```python
from build123d import *

# Parameters (mm, degrees)
SKETCH1_W                        = 63.5
SKETCH1_H                        = 12.7
BOSS_EXTRUDE1_DEPTH              = 50.8
F_25_0_1495_DIAMETER_HOLE1_D     = 3.7973
F_25_0_1495_DIAMETER_HOLE1_DEPTH = 12.7
F_25_0_1495_DIAMETER_HOLE1_TIP   = 1.140824014
F_7_0_201_DIAMETER_HOLE1_D       = 5.1054
F_7_0_201_DIAMETER_HOLE1_DEPTH   = 12.7
F_7_0_201_DIAMETER_HOLE1_TIP     = 1.533816902


with BuildPart() as part:
    # Sketch1 → Boss-Extrude1 (new body)
    with BuildSketch(Plane(origin=(0, 0, 0), x_dir=(1, 0, 0), z_dir=(0, 1, 0))):
        with Locations((31.75, 6.35)):
            Rectangle(SKETCH1_W, SKETCH1_H)
    extrude(amount=BOSS_EXTRUDE1_DEPTH)

    # #25 (0.1495) Diameter Hole1
    with Locations(Plane(origin=(0, 50.8, 0), x_dir=(1, 0, 0), z_dir=(0, 1, 0))):
        with Locations((6.35, 6.35), (57.15, 6.35)):
            Hole(F_25_0_1495_DIAMETER_HOLE1_D / 2, depth=F_25_0_1495_DIAMETER_HOLE1_DEPTH)
            with Locations((0, 0, -(F_25_0_1495_DIAMETER_HOLE1_DEPTH + F_25_0_1495_DIAMETER_HOLE1_TIP / 2))):  # 118° drill point
                Cone(0, F_25_0_1495_DIAMETER_HOLE1_D / 2, F_25_0_1495_DIAMETER_HOLE1_TIP, mode=Mode.SUBTRACT)

    # #7 (0.201) Diameter Hole1
    with Locations(Plane(origin=(0, 0, -12.7), x_dir=(-1, 0, 0), z_dir=(0, 0, -1))):
        with Locations((-22.225, 43.18), (-41.275, 43.18)):
            Hole(F_7_0_201_DIAMETER_HOLE1_D / 2, depth=F_7_0_201_DIAMETER_HOLE1_DEPTH)
            with Locations((0, 0, -(F_7_0_201_DIAMETER_HOLE1_DEPTH + F_7_0_201_DIAMETER_HOLE1_TIP / 2))):  # 118° drill point
                Cone(0, F_7_0_201_DIAMETER_HOLE1_D / 2, F_7_0_201_DIAMETER_HOLE1_TIP, mode=Mode.SUBTRACT)


solid = part.part
```
Model file for the job. Use its own axes, mm. Coordinates: 2 decimals unless noted, no trailing zeros. Write each loop counter-clockwise with the first axis right and the second up, starting at its lowest first coordinate (ties: lowest second). Pieces come first, ordered by that corner, then holes. Notation, with made-up numbers: (32, 75.25) - (44, 75.25) arc R23 ccw to (44, 102.25) - close; hole circle Ø6 at (-14, 2.25). An arc over 180 degrees is marked (long way). One line per question, with ' | ' between items. Start each with the question number.
Q1. Pull direction X, two halves, no side cores. Call faces 1 (the face through (55.34, 44.36, -6.92)), 2 (the face through (31, 25, -12.7)), 3 (the face through (7.857, 44.361, -5.195)), 4 (the face through (0, 25, -6)): pulls with the +X half, pulls with the -X half, needs draft (parallel to the pull), parting line crosses it, or undercut.
Q2. Drill centre lines: line 1 (X direction, y = 43.18, z = -8.75); line 2 (X direction, y = 45, z = -6.5); line 3 (Z direction, x = 57.15, y = 47.5). Where is each one in solid material? Low to high. Write a range as [from, to].
Q3. Pin check, flat tips, straight feed: pin 1 (3 mm diameter, centred on y = 16, z = -4, fed in from -X); pin 2 (2.5 mm diameter, centred on x = 6.35, z = -6.35, fed in from +Y); pin 3 (3 mm diameter, centred on x = 22.225, y = 43.18, fed in from -Z). Stop position of each tip, or through.
Q4. Cut at A-A, the plane y = 43.18. List the corners of the cut face in (x, z).
Answer below:
1) face 1: undercut | face 2: needs draft | face 3: undercut | face 4: pulls with the -X half
2) line 1: [0, 19.67], [24.78, 38.72], [43.83, 63.5] | line 2: [0, 4.46], [8.24, 20.44], [24.01, 39.49], [43.06, 55.26], [59.04, 63.5] | line 3: [-12.7, -8.25], [-4.45, 0]
3) pin 1: x = 0 | pin 2: y = 37.71 | pin 3: through
4) outline: (0, -12.7) - (19.67, -12.7) - (19.67, 0) - (0, 0) - close; (24.78, -12.7) - (38.72, -12.7) - (38.72, 0) - (24.78, 0) - close; (43.83, -12.7) - (63.5, -12.7) - (63.5, 0) - (43.83, 0) - close; hole circle Ø3.8 at (6.35, -6.35); hole circle Ø3.8 at (57.15, -6.35)
